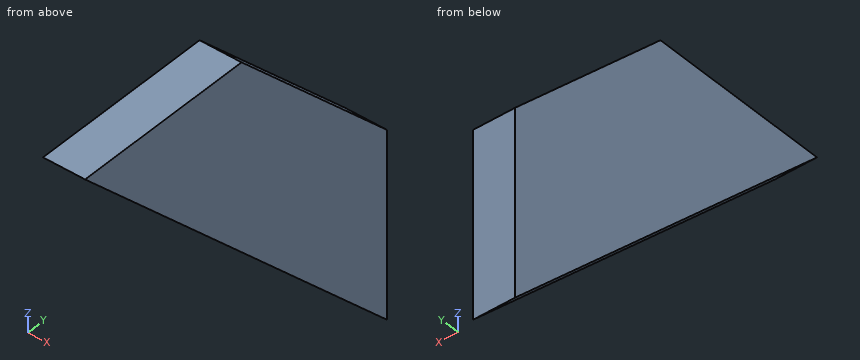
Autodesk Inventor part; units mm, degrees
ref_plane "YZ Plane" through (0, 0, 0) normal (1, 0, 0) x (0, 1, 0)
ref_plane "XZ Plane" through (0, 0, 0) normal (0, 1, 0) x (-1, 0, 0)
ref_plane "XY Plane" through (0, 0, 0) normal (0, 0, 1) x (1, 0, 0)
sketch "Sketch1" plane through (0, 0, 0) normal (1, 0, 0) x (0, 1, 0)
  line L0 (0, 0) -> (215.5261, -215.5261)
  line L1 (0, 0) -> (304.8, 0) construction
  line L2 (381, -183.4344) -> (337.2656, -139.7)
  line L3 (337.2656, -139.7) -> (197.5656, 0)
  line L4 (197.5656, 0) -> (0, 0)
  line L5 (215.5261, -215.5261) -> (381, -381)
  line L6 (381, -183.4344) -> (381, -381)
  dimension "d0" = 304.8
  dimension "d1" = 45
  dimension "d2" = 139.7
  dimension "d5" = 381
extrude "Extrusion1" add sketch "Sketch1" along normal blind 44.45
properties part number "gableSupport" material "Wood (Birch)"
Verification items for the finished model (mm, model axes). Coordinates: 2 decimals unless noted, no trailing zeros. Order: outer loops, then holes, each group sorted by start corner. A loop starts at its lowest first (then second) coordinate and runs counter-clockwise, first axis right, second up.
Item 1: Material ranges on L1, parallel to Y at x = 22.5, z = -203; L2, parallel to Y at x = 15, z = -259.5; L3, parallel to Z at x = 13.5, y = 52, recorded low to high.
Filled in:
L1: y = 203 to 381
L2: y = 259.5 to 381
L3: z = -52 to 0
Item 2: Section check B-B, the plane y = 101. Enter the section's corners in (x, z).
Filled in:
outline: (0, -101) - (44.45, -101) - (44.45, 0) - (0, 0) - close
Item 3: Depth check by flat-ended pin: pin 1 (4 mm diameter, centred on x = 33, z = -86.5, fed in from +Y); pin 2 (6 mm diameter, centred on x = 35, y = 243.5, fed in from -Z); pin 3 (8 mm diameter, centred on x = 37.5, z = -80.5, fed in from +Y). Enter the tip coordinate at first touch or a pass-through.
Filled in:
pin 1: stops at y = 286.07
pin 2: stops at z = -246.5
pin 3: stops at y = 282.07
Item 4: Section check A-A, the plane x = 14. Enter the section's corners in (y, z), then the cut area to 3 significant figures.
Filled in:
outline: (0, 0) - (381, -381) - (381, -183.43) - (197.57, 0) - close
area: 55,800 mm2
